Build history of the part. All positions in model axes, mm. Face numbers are marked on the shaded views. A direction names the side the tool comes from. Round coordinates to 2 decimals unless told otherwise and drop trailing zeros. Write each loop counter-clockwise with the first axis right and the second up, starting at its lowest first coordinate (ties: lowest second). Pieces come first, ordered by that corner, then holes. Notation, with made-up numbers: M -3.5,-19 L 55.5,-19 A20 cw 55.5,15 Z; hole C 42,17 d1. An arc over 180 degrees is marked long. One line per item, written item: value. Start each with the question number.
Autodesk Inventor part; units mm, degrees
ref_plane "YZ Plane" through (0, 0, 0) normal (1, 0, 0) x (0, 1, 0)
ref_plane "XZ Plane" through (0, 0, 0) normal (0, 1, 0) x (-1, 0, 0)
ref_plane "XY Plane" through (0, 0, 0) normal (0, 0, 1) x (1, 0, 0)
sketch "Sketch1" plane through (0, 0, 0) normal (0, 1, 0) x (-1, 0, 0)
  circle A0 centre (0, 0) radius 12.5
  line L0 (0, 0) -> (7.75, 0) construction
  circle A1 centre (5.4801, -5.4801) radius 2
  circle A2 centre (-5.4801, -5.4801) radius 2
  circle A3 centre (-5.4801, 5.4801) radius 2
  circle A4 centre (5.4801, 5.4801) radius 2
  circle A5 centre (0, -7.75) radius 2
  circle A6 centre (0, 7.75) radius 2
  dimension "d0" = 25
  dimension "d3" = 4
  dimension "d6" = 360
  dimension "d8" = 4
  dimension "d11" = 360
extrude "Extrusion1" add sketch "Sketch1" along normal blind 5
sketch "Sketch2" plane through (0, 5, 0) normal (0, 1, 0) x (1, 0, 0)
  line L0 (4.991, -3.5408) -> (4.991, 3.5408)
  line L1 (-66.4503, 5) -> (-66.4503, -5)
  line L2 (4.991, -4.9385) -> (14.991, -4.9385) construction
  line L3 (-82.7386, 0) -> (31.2793, 0)
  arc A0 (-3.5548, -4.9385) -> (-7.4216, -5) centre (-5.4801, -5.4801) ccw
  line L4 (-66.4503, -5) -> (-7.4216, -5)
  line L5 (-3.5548, -4.9385) -> (3.5548, -4.9385)
  circle A1 centre (-5.4801, 5.4801) radius 2
  arc A2 (-7.4216, 5) -> (-3.5497, 4.9571) centre (-5.4801, 5.4801) ccw
  line L6 (3.5497, 4.9571) -> (-3.5497, 4.9571)
  line L7 (-7.4216, 5) -> (-66.4503, 5)
  arc A3 (4.991, -3.5408) -> (3.5548, -4.9385) centre (5.4801, -5.4801) ccw
  circle A4 centre (5.4801, 5.4801) radius 2
  arc A5 (3.5497, 4.9571) -> (4.991, 3.5408) centre (5.4801, 5.4801) ccw
  dimension "d24" = 10
  dimension "d25" = 90
  dimension "d26" = 70
  dimension "d27" = 4
  dimension "d28" = 4
  dimension "d29" = 4
  dimension "d30" = 4
extrude "Extrusion2" add sketch "Sketch2" along normal blind 5 contours A3 L5 A0 L4 L1 L3 L0 | L3 L1 L7 A1 L6 A4 L0
sketch "Sketch4" plane through (0, 10, 0) normal (0, 1, 0) x (1, 0, 0)
  line L0 (-3.5548, -4.9385) -> (3.5548, -4.9385)
  line L1 (-3.5548, -4.9385) -> (3.5548, -4.9385)
  line L2 (3.5497, 4.9571) -> (-3.5497, 4.9571)
  line L3 (-3.5497, 4.9571) -> (3.5497, 4.9571)
  line L4 (-4.4956, -10.2074) -> (2.6201, -10.2074)
  point P0 (0, 0)
sketch "Sketch8" plane through (0, 5, 0) normal (0, 1, 0) x (1, 0, 0)
  circle A0 centre (-5.4801, 5.4801) radius 2
  circle A1 centre (-5.4801, 5.4801) radius 3
  circle A2 centre (-5.4801, -5.4801) radius 2
  circle A3 centre (-5.4801, -5.4801) radius 3
  circle A4 centre (5.4801, 5.4801) radius 2
  circle A5 centre (5.4801, 5.4801) radius 3
  arc A6 (3.5548, -4.9385) -> (4.991, -3.5408) centre (5.4801, -5.4801) ccw
  circle A7 centre (5.4801, -5.4801) radius 3
  point P0 (0, 0)
  dimension "d50" = 6
  dimension "d51" = 6
  dimension "d52" = 6
  dimension "d53" = 6
extrude "Extrusion6" cut sketch "Sketch8" along normal blind 39.25 contours A0 | A1 | A2 | A3 | A4 | A5 | A7
sketch "Sketch33" plane through (0, 10, 0) normal (0, 1, 0) x (1, 0, 0)
  line L0 (-2.5294, -4.9385) -> (2.5294, -4.9385)
  arc A0 (-8.4414, 5) -> (-2.526, 4.9571) centre (-5.4801, 5.4801) ccw
  line L1 (-2.5294, -4.9385) -> (-2.526, 4.9571)
  line L2 (-2.526, 4.9571) -> (-2.526, 4.9571)
  line L3 (2.526, 4.9571) -> (-2.526, 4.9571)
  line L4 (-2.526, 4.9571) -> (-2.5215, 18.4671)
  line L5 (-2.5215, 18.4671) -> (-2.534, -18.5329)
  point P0 (0, 0)
  dimension "d105" = 13.51
  dimension "d106" = 37
sketch "Sketch34" plane through (-66.4503, 5, -5) normal (-1, 0, 0) x (0, 0, 1)
  point P0 (5, -5)
properties part number "US holder1"
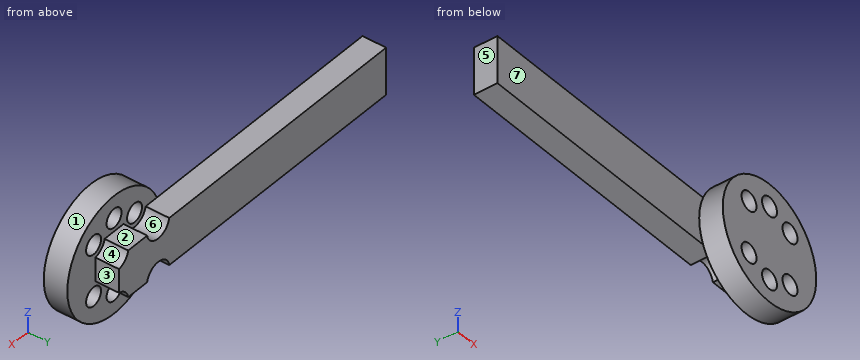
Item 1: Drill centre lines: line 1 (Z direction, x = 0, y = 2.7); line 2 (X direction, y = 6.25, z = -3.25); line 3 (X direction, y = 4, z = -6.5). Where is each one in solid material? Low to high.
Item 2: Two-plate mould, pull along X, no slides. Class the marked faces 4, 5, 6 and 7: pulls with the +X half, pulls with the -X half, needs draft (parallel to the pull), parting line crosses it, or undercut.
Item 3: Drop flat-ended pins along their axis: pin 1 (4 mm diameter, centred on x = -40.5, y = 8, fed in from -Z); pin 2 (1 mm diameter, centred on x = -14, z = 3.5, fed in from -Y); pin 3 (4.5 mm diameter, centred on x = 0, z = 7.75, fed in from +Y). Give the stop position or say it passes through.
Item 4: Cut at D-D, the plane z = -8.5. Write the cut outline in (x, y).
Item 5: Cut at B-B, the plane z = 0. Write the cut outline in (x, y).
Item 6: Which spindle directions (+Z, -Z, +X, -X, +Y, -Y) get a long thin tool onto all of the face, cutting with end or side? Do the marked faces 1, 2 and 3. Say none if no direction does.
Item 7: Cut at C-C, the plane y = 6.5. Write the cut outline in (x, z).
Item 8: Cut at A-A, the plane x = 0. Write the cut outline in (y, z).
Computed values:
1. line 1: z = -12.5 to -9.75, -5.75 to 5.75, 9.75 to 12.5
1. line 2: x = -66.45 to -7.49, -3.47 to 3.47
1. line 3: x = -10.68 to -7.2, -3.76 to -1.56, 1.56 to 3.76, 7.2 to 10.68
2. face 4: pulls with the +X half
2. face 5: pulls with the -X half
2. face 6: undercut
2. face 7: needs draft
3. pin 1: stops at z = -5
3. pin 2: stops at y = 5
3. pin 3: stops at y = 5
4. outline: M -9.17,0 L -1.85,0 L -1.85,5 L -9.17,5 Z; M 1.85,0 L 9.17,0 L 9.17,5 L 1.85,5 Z
5. outline: M -66.45,5 L -12.5,5 L -12.5,0 L 12.5,0 L 12.5,5 L 4.99,5 L 4.99,10 L -66.45,10 Z
6. face 1: -Y
6. face 2: +Z, +X, +Y
6. face 3: +Z, -Z, +X, +Y
7. outline: M -66.45,-5 L -8.44,-5 A3 cw -2.53,-4.96 L 2.53,-4.96 A3 cw 4.99,-2.52 L 4.99,2.52 A3 cw 2.53,4.94 L -2.53,4.94 A3 cw -8.44,5 L -66.45,5 Z
8. outline: M 0,-12.5 L 5,-12.5 L 5,-9.75 L 0,-9.75 Z; M 0,-5.75 L 5,-5.75 L 5,-4.96 L 10,-4.96 L 10,4.94 L 5,4.94 L 5,5.75 L 0,5.75 Z; M 0,9.75 L 5,9.75 L 5,12.5 L 0,12.5 Z
